Build history of the part. All positions in model axes, mm. Round coordinates to 2 decimals unless told otherwise and drop trailing zeros. Loops run counter-clockwise (first coordinate to the right, second up) from the corner with the lowest first, then second, coordinate; pieces in that order, holes last. Notation, with made-up numbers: M -17.75,81.25 L 10.25,81.25 A16 ccw 10.25,93.25 Z; hole C 63.5,31 d1. An arc over 180 degrees is marked long. One line per item, written item: value.
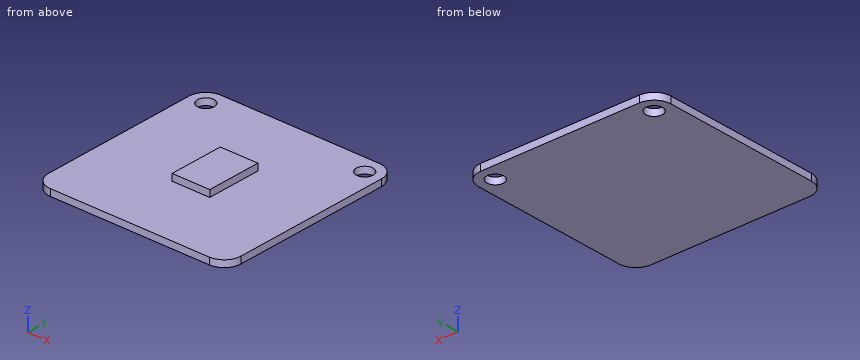
Autodesk Inventor part; units mm, degrees
ref_plane "YZ Plane" through (0, 0, 0) normal (1, 0, 0) x (0, 1, 0)
ref_plane "XZ Plane" through (0, 0, 0) normal (0, 1, 0) x (-1, 0, 0)
ref_plane "XY Plane" through (0, 0, 0) normal (0, 0, 1) x (1, 0, 0)
sketch "Sketch1" plane through (0, 0, 0) normal (0, 0, 1) x (1, 0, 0)
  line L0 (-10.7511, 9.0038) -> (12.2489, 9.0038)
  line L1 (12.2489, 9.0038) -> (12.2489, -13.9962)
  line L2 (12.2489, -13.9962) -> (-10.7511, -13.9962)
  line L3 (-10.7511, -13.9962) -> (-10.7511, 9.0038)
  point P0 (0, 0)
  dimension "d0" = 23
  dimension "d1" = 23
extrude "Extrusion1" add sketch "Sketch1" along normal blind 0.8
fillet "Fillet1" radius 2 4 edges at (12.2489, 9.0038, 0.4) (-10.7511, 9.0038, 0.4) (12.2489, -13.9962, 0.4) (-10.7511, -13.9962, 0.4)
sketch "Sketch2" plane through (0, 0, 0.8) normal (0, 0, 1) x (1, 0, 0)
  arc A0 (-8.7511, 9.0038) -> (-10.7511, 7.0038) centre (-8.7511, 7.0038) ccw
  circle A1 centre (-8.7511, 7.0038) radius 1
  arc A2 (12.2489, 7.0038) -> (10.2489, 9.0038) centre (10.2489, 7.0038) ccw
  circle A3 centre (10.2489, 7.0038) radius 1
  point P0 (0, 0)
  dimension "d5" = 2
  dimension "d6" = 2
extrude "Extrusion2" cut sketch "Sketch2" against normal blind 0.8
sketch "Sketch3" plane through (0, 0, 0.8) normal (0, 0, 1) x (1, 0, 0)
  line L0 (10.2489, 9.0038) -> (-8.7511, 9.0038)
  line L1 (-8.7511, -13.9962) -> (10.2489, -13.9962)
  line L2 (0.7489, 9.0038) -> (10.2489, 9.0038)
  line L3 (10.2489, 9.0038) -> (10.2489, -13.9962)
  line L4 (10.2489, -13.9962) -> (0.7489, -13.9962)
  line L5 (0.7489, -13.9962) -> (0.7489, 9.0038)
  line L6 (2.9989, -5.7462) -> (-1.5011, -5.7462)
  line L7 (-1.5011, -5.7462) -> (-1.5011, 0.7538)
  line L8 (-1.5011, 0.7538) -> (2.9989, 0.7538)
  line L9 (2.9989, 0.7538) -> (2.9989, -5.7462)
  line L10 (2.9989, -5.7462) -> (-1.5011, 0.7538) construction
  line L11 (-1.5011, -5.7462) -> (2.9989, 0.7538) construction
  point P0 (0, 0)
  point P1 (0.7489, -2.4962)
  dimension "d9" = 4.5
  dimension "d10" = 6.5
extrude "Extrusion3" add sketch "Sketch3" along normal blind 0.8 contours L8 L9 L6 L5 | L5 L6 L7 L8
properties part number "Encoder"
Item 1: Drop flat-ended pins along their axis: P1, Ø0.6, axis at x = -0.5, z = 1.5, coming from the +Y side; P2, Ø1.2, axis at x = 10.25, y = 7, coming from the -Z side; P3, Ø2, axis at x = -3.5, y = -11.5, coming from the +Z side. Give the stop position or say it passes through.
Check values:
P1: stops at y = 0.75
P2: passes through
P3: stops at z = 0.8
Item 2: Slice it at A-A, the plane z = 0.4. Give the cut face in (x, y), and give its area (3 significant figures).
Check values:
outline: M -10.75,-12 A2 ccw -8.75,-14 L 10.25,-14 A2 ccw 12.25,-12 L 12.25,7 A2 ccw 10.25,9 L -8.75,9 A2 ccw -10.75,7 Z; hole C -8.75,7 d2; hole C 10.25,7 d2
area: 519 mm2
Item 3: Slice it at B-B, the plane y = -3.75. Give the cut face in (x, z), and give its area (3 significant figures).
Check values:
outline: M -10.75,0 L 12.25,0 L 12.25,0.8 L 3,0.8 L 3,1.6 L -1.5,1.6 L -1.5,0.8 L -10.75,0.8 Z
area: 22.0 mm2
Item 4: Wall check: line 1 along Z through (x, y) = (4, -11.5); line 2 along X through (y, z) = (-3.5, 1.1). Give the ranges that are in metal, low to high.
Check values:
line 1: z = 0 to 0.8
line 2: x = -1.5 to 3
Item 5: Slice it at D-D, the plane y = -9.5. Give the cut face in (x, z), and give its area (3 significant figures).
Check values:
outline: M -10.75,0 L 12.25,0 L 12.25,0.8 L -10.75,0.8 Z
area: 18.4 mm2
Item 6: Slice it at C-C, the plane x = -3.5. Give the cut face in (y, z), and give its area (3 significant figures).
Check values:
outline: M -14,0 L 9,0 L 9,0.8 L -14,0.8 Z
area: 18.4 mm2
